Read the model definition and answer for the solid it produces. Units are mm, in the model's axes. A direction names the side the tool comes from. Give positions to 0.01 mm unless a question says otherwise; leave off trailing zeros. Order: outer loops, then holes, each group sorted by start corner. A loop starts at its lowest first (then second) coordinate and runs counter-clockwise, first axis right, second up.
Item 1: A cutting plane is placed at A-A (z = 0). Write down the section's boundary in (x, y), plus the area to 3 significant figures.
Item 2: Given pin 1 Ø5 at (x, y) = (13, 43) entering from -Z; pin 2 Ø3 at (x, y) = (-4, 15) entering from +Z; pin 3 Ø5 at (x, y) = (8.5, 29.5) entering from -Z, each flat-ended and moving along its own axis, determine where each tip first touches the part or whether it passes through.
Item 3: A cutting plane is placed at B-B (x = -1). Write down the section's boundary in (y, z), plus the area to 3 significant figures.
Item 4: A cutting plane is placed at D-D (x = 22). Write down the section's boundary in (y, z), plus the area to 3 significant figures.
Item 5: Find the intervals of material crossed by line 1 along Y through (x, z) = (-25, 10); line 2 along Z through (x, y) = (12.5, 23); line 3 along Z through (x, y) = (20, 26), in increasing order.
Item 6: The mould has two halves that part along Z. Classify faces 1 (the face through (13, 20, 0)), 2 (the face through (-26.474, 34.65, -1.165)), 3 (the face through (12.8, 10, -23.5)): +Z half, -Z half, draft (parallel to the pull), parting line (faces both ways), or undercut.
Item 7: Which of the six approach directions +Z, -Z, +X, -X, +Y, -Y give full straight-line access (tool end or side, diameter ignored) to faces 4 (the face through (0, 40, 0)), 5 (the face through (-28, 5, 21))?
Item 8: A cutting plane is placed at C-C (y = 41). Write down the section's boundary in (x, z).
from build123d import *

# Parameters (mm, degrees)
CROQUIS1_R              = 35
SALIENTE_EXTRUIR1_DEPTH = 10
CROQUIS2_R              = 26.5
SALIENTE_EXTRUIR3_DEPTH = 50
CROQUIS4_W              = 20
CROQUIS4_H              = 40
CORTAR_EXTRUIR2_DEPTH   = 40


with BuildPart() as part:
    # Croquis1 → Saliente-Extruir1 (new body)
    with BuildSketch(Plane(origin=(0, 0, 0), x_dir=(1, 0, 0), z_dir=(0, 1, 0))):
        Circle(CROQUIS1_R)
    extrude(amount=SALIENTE_EXTRUIR1_DEPTH)

    # Croquis2 → Saliente-Extruir3 (add)
    with BuildSketch(Plane(origin=(0, 10, 0), x_dir=(1, 0, 0), z_dir=(0, 1, 0))):
        Circle(CROQUIS2_R)
    extrude(amount=SALIENTE_EXTRUIR3_DEPTH)

    # Croquis4 → Cortar-Extruir2 (cut)
    with BuildSketch(Plane(origin=(0, 0, 0), x_dir=(0, 0, -1), z_dir=(1, 0, 0))):
        with Locations((0, 40)):
            Rectangle(CROQUIS4_W, CROQUIS4_H)
    extrude(amount=CORTAR_EXTRUIR2_DEPTH, mode=Mode.SUBTRACT)


solid = part.part
Response values:
1. outline: (-35, 0) - (35, 0) - (35, 10) - (26.5, 10) - (26.5, 20) - (0, 20) - (0, 60) - (-26.5, 60) - (-26.5, 10) - (-35, 10) - close
1. area: 2,290 mm2
2. pin 1: stops at z = -24.33
2. pin 2: stops at z = 26.38
2. pin 3: stops at z = -25.81
3. outline: (0, -34.99) - (10, -34.99) - (10, -26.48) - (60, -26.48) - (60, 26.48) - (10, 26.48) - (10, 34.99) - (0, 34.99) - close
3. area: 3,350 mm2
4. outline: (0, -27.22) - (10, -27.22) - (10, -14.77) - (60, -14.77) - (60, -10) - (20, -10) - (20, 10) - (60, 10) - (60, 14.77) - (10, 14.77) - (10, 27.22) - (0, 27.22) - close
4. area: 1,220 mm2
5. line 1: y = 0 to 10
5. line 2: z = -23.37 to -10, 10 to 23.37
5. line 3: z = -17.39 to -10, 10 to 17.39
6. face 1: undercut
6. face 2: parting line
6. face 3: draft
7. face 4: +X, +Y
7. face 5: +Y, -Y
8. outline: (0, -10) - (0, 10) - (24.54, 10) arc R26.5 ccw (long way) to (24.54, -10) - close
